Geometry: final body of the model. Coordinates: model frame, mm. A direction names the side the tool comes from. Give positions to 0.01 mm unless a question says otherwise; leave off trailing zeros. Write each loop counter-clockwise with the first axis right and the second up, starting at its lowest first coordinate (ties: lowest second). Pieces come first, ordered by that corner, then holes. Notation, with made-up numbers: (-36.75, 84.5) -> (-9.75, 84.5) arc R17 cw to (-9.75, 117.5) -> close; hole circle Ø1 at (-6, 21). An arc over 180 degrees is marked (long way). Answer as a JSON object with one key per item and string values.
from build123d import *

# Parameters (mm, degrees)
EXTRUDE_1_DEPTH     = 30
SKETCH_2_R          = 4
CUT_EXTRUDE_1_DEPTH = 31
CUT_EXTRUDE_4_DEPTH = 30
SKETCH1_W           = 30
SKETCH1_H           = 30
BOSS_EXTRUDE1_DEPTH = 27
CHAMFER1_SIZE       = 30
CHAMFER1_SIZE2      = 17.320508076
CHAMFER2_SIZE       = 1
CHAMFER2_SIZE2      = 1.191753593


with BuildPart() as part:
    # Эскиз1 → Бобышка-Вытянуть1 (new body)
    with BuildSketch(Plane(origin=(0, 0, 0), x_dir=(1, 0, 0), z_dir=(0, 1, 0))):
        Polygon((-20, -15), (-35, -15), (-35, 15), (-20, 15), (20, 15), (20, -15), align=None)
    extrude(amount=EXTRUDE_1_DEPTH)

    # Эскиз2 → Вырез-Вытянуть1 (cut, through all)
    with BuildSketch(Plane(origin=(0, 30, 0), x_dir=(1, 0, 0), z_dir=(0, 1, 0))):
        with Locations(Location((-20, 0, 0), (0, 0, 270))):  # turned: the seam where the file's is
            Circle(SKETCH_2_R)
    extrude(amount=-CUT_EXTRUDE_1_DEPTH, mode=Mode.SUBTRACT)

    # Эскиз5 → Вырез-Вытянуть4 (cut)
    with BuildSketch(Plane(origin=(20, 0, 0), x_dir=(0, 0, -1), z_dir=(1, 0, 0))):
        Polygon((4.458832066, 4.601018482), (11.015265685, 12.414671802), (-4.458832066, 25.398981518), (-11.015265685, 17.585328198), align=None)
    extrude(amount=-CUT_EXTRUDE_4_DEPTH, mode=Mode.SUBTRACT)

    # Sketch1 → Boss-Extrude1 (add)
    with BuildSketch(Plane.ZY.offset(35)):
        with Locations((0, 15)):
            Rectangle(SKETCH1_W, SKETCH1_H)
    extrude(amount=BOSS_EXTRUDE1_DEPTH)

    # Chamfer1
    chamfer1_edges = [part.edges().sort_by_distance(p)[0] for p in [
        (-62, 15, -15),
    ]]
    chamfer1_side = [part.faces().sort_by_distance(p)[0] for p in [
        (-21, 15, -15),
    ]]
    chamfer(chamfer1_edges, length=CHAMFER1_SIZE, length2=CHAMFER1_SIZE2, reference=chamfer1_side[0])

    # Chamfer2
    chamfer2_edges = [part.edges().sort_by_distance(p)[0] for p in [
        (20, 18.90682666, -3.278216809),
        (20, 21.492154858, 7.737048876),
        (20, 11.09317334, 3.278216809),
        (20, 8.507845142, -7.737048876),
    ]]
    chamfer2_side = [part.faces().sort_by_distance(p)[0] for p in [
        (20, 15, -14.575735931),
    ]]
    chamfer(chamfer2_edges, length=CHAMFER2_SIZE, length2=CHAMFER2_SIZE2, reference=chamfer2_side[0])


solid = part.part
Q1. Mould query, pull axis Y, two halves, no side actions, for faces 3 (the flat face through (-11, 0, 0)), 4 (the flat face through (-11, 30, 0)), 5 (the flat face through (-20, 15, 15)), 6 (the flat face through (19.4, 10.8, 3.7)). Classes: pulls with the +Y half, pulls with the -Y half, needs draft (parallel to the pull), parting line crosses it, or undercut.
Values:
{"face 3": "pulls with the -Y half", "face 4": "pulls with the +Y half", "face 5": "needs draft", "face 6": "undercut"}
Q2. Cut plane B-B (x = 2.5). Return the cut outline in (y, z), and give its area (3 significant figures).
Values:
{"outline": "(0, -15) -> (30, -15) -> (30, 15) -> (0, 15) -> close; hole (4.6, -4.46) -> (12.41, -11.02) -> (25.4, 4.46) -> (17.59, 11.02) -> close", "area": "694 mm²"}
Q3. Cut plane D-D (z = 7.5). Return the cut outline in (x, y).
Values:
{"outline": "(-62, 0) -> (20, 0) -> (20, 13.33) -> (18.81, 14.64) -> (-10, 14.64) -> (-10, 21.77) -> (18.81, 21.77) -> (20, 23.33) -> (20, 30) -> (-62, 30) -> close"}
Q4. Set-up query: faces 1 (the flat face through (19.396, 8.126, -8.06)), 2 (the cylindrical face through (-16.034, 15.21, -0.521)). Return all of +Z, -Z, +X, -X, +Y, -Y with unobstructed straight access to the full face (end or side cutting, diameter ignored); none if empty.
Values:
{"face 1": "+X", "face 2": "+Y, -Y"}
Q5. First-contact query: P1, Ø5, axis at x = -47, y = 6, coming from the -Z side; P2, Ø8, axis at x = -45.5, y = 18.5, coming from the -Z side; P3, Ø3, axis at x = -36.5, y = 21.5, coming from the -Z side. Flat tips, straight axial feed; report the tip coordinate or a pass-through.
Values:
{"P1": "z = -7.78", "P2": "z = -9.52", "P3": "z = -13.27"}
Q6. Cut plane A-A (x = -20). Return the cut outline in (y, z), and give its area (3 significant figures).
Values:
{"outline": "(0, -15) -> (30, -15) -> (30, -4) -> (0, -4) -> close; (0, 4) -> (30, 4) -> (30, 15) -> (0, 15) -> close", "area": "660 mm²"}
Q7. Cut plane C-C (y = 14.5). Return the cut outline in (x, z), and give its area (3 significant figures).
Values:
{"outline": "(-62, 2.32) -> (-32, -15) -> (20, -15) -> (20, -10.09) -> (18.81, -8.53) -> (-10, -8.53) -> (-10, 7.34) -> (18.81, 7.34) -> (20, 8.89) -> (20, 15) -> (-62, 15) -> close; hole circle Ø8 at (-20, 0)", "area": "1,670 mm²"}
Q8. Material intervals for L1, parallel to Z at x = 12, y = 14; L2, parallel to X at y = 14.5, z = 2.5; L3, parallel to Y at x = 7, z = -9.75, sorted ascending. Write a range as from..to.
Values:
{"L1": "-15..-9.13, 6.74..15", "L2": "-62..-23.12, -16.88..-10", "L3": "0..10.91, 13.48..30"}
